Can you work these out from the drawing? Everything is in mm from the part's minimum corner. Round coordinates to 2 decimals unless told otherwise and drop trailing zeros. Order: outer loops, then holes, each group sorted by start corner. A loop starts at its lowest first (then second) coordinate and runs counter-clockwise, first axis right, second up. Notation, with made-up numbers: (88, 28.25) -> (133, 28.25) arc R27 cw to (133, 49.25) -> close; hole circle Ø7 at (-24, 46). An arc over 180 degrees is marked (long way). One line per item, written item: value.
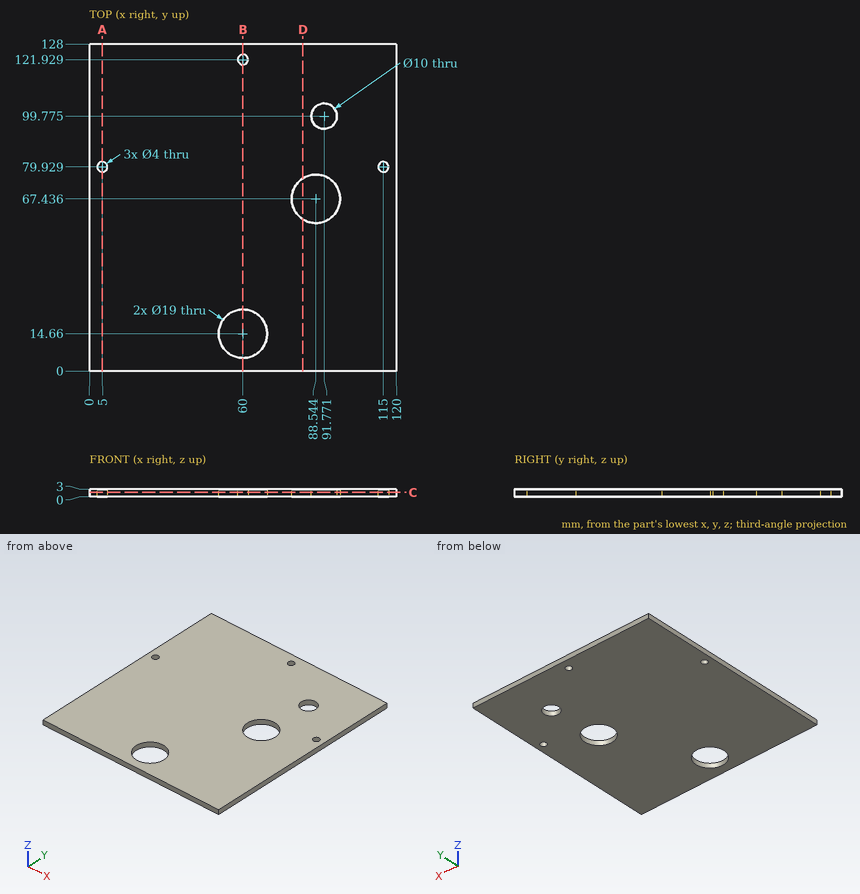
Q1. Will this pin go through, and if not, where does the flat tip stop? pin 1 Ø15 at (x, y) = (60, 14.66) entering from -Z.
Answers below:
pin 1: through
Q2. I want a section at C-C on z = 1.8. List the corners of the cut face in (x, y) for me (1 decimal).
Answers below:
outline: (0, 0) -> (120, 0) -> (120, 128) -> (0, 128) -> close; hole circle Ø4 at (5, 79.9); hole circle Ø19 at (60, 14.7); hole circle Ø4 at (60, 121.9); hole circle Ø19 at (88.5, 67.4); hole circle Ø10 at (91.8, 99.8); hole circle Ø4 at (115, 79.9)
Q3. I want a section at B-B on x = 60. List the corners of the cut face in (y, z) for me, plus the area to 3 significant figures.
Answers below:
outline: (0, 0) -> (5.16, 0) -> (5.16, 3) -> (0, 3) -> close; (24.16, 0) -> (119.93, 0) -> (119.93, 3) -> (24.16, 3) -> close; (123.93, 0) -> (128, 0) -> (128, 3) -> (123.93, 3) -> close
area: 315 mm^2
Q4. Please list where these lines run through material, in increasing order: line 1 along X through (y, z) = (15, 2.1); line 2 along X through (y, z) = (60, 2.5) (1 decimal); line 3 along Y through (x, z) = (5, 0.65).
Answers below:
line 1: 0 to 50.51, 69.49 to 120
line 2: 0 to 82.6, 94.5 to 120
line 3: 0 to 77.93, 81.93 to 128
Q5. I want a section at A-A on x = 5. List the corners of the cut face in (y, z) for me.
Answers below:
outline: (0, 0) -> (77.93, 0) -> (77.93, 3) -> (0, 3) -> close; (81.93, 0) -> (128, 0) -> (128, 3) -> (81.93, 3) -> close
Q6. I want a section at D-D on x = 83.5. List the corners of the cut face in (y, z) for me (1 decimal), plus the area to 3 significant figures.
Answers below:
outline: (0, 0) -> (59.4, 0) -> (59.4, 3) -> (0, 3) -> close; (75.5, 0) -> (128, 0) -> (128, 3) -> (75.5, 3) -> close
area: 336 mm^2
